Verification items for the finished model (mm, model axes). Round coordinates to 2 decimals unless told otherwise and drop trailing zeros. Loops run counter-clockwise (first coordinate to the right, second up) from the corner with the lowest first, then second, coordinate; pieces in that order, holes last. Notation, with made-up numbers: M -31,8.5 L 6,8.5 A20 cw 6,12.5 Z; hole C 22.5,36.25 d9. An arc over 180 degrees is marked long. One line per item, written item: value.
from build123d import *

# Parameters (mm, degrees)
F0_W     = 50
F0_H     = 20
F1_DEPTH = 114
F3_D     = 5
F3_DEPTH = 20.6
F3_TIP   = 1.5021515476
F5_D     = 10
F5_DEPTH = 42
F5_TIP   = 3.0043030951
F6_R     = 2


with BuildPart() as f1:
    # F0 (on Top) → F1 (new body)
    with BuildSketch(Plane.XY):
        Rectangle(F0_W, F0_H)
    extrude(amount=F1_DEPTH)

    # F3
    with Locations(Plane.XY.offset(114)):
        with Locations((-15, 0), (15, 0)):
            Hole(F3_D / 2, depth=F3_DEPTH)
            with Locations((0, 0, -(F3_DEPTH + F3_TIP / 2))):  # 118° drill point
                Cone(0, F3_D / 2, F3_TIP, mode=Mode.SUBTRACT)

    # F5
    with Locations(Plane(origin=(0, 0, 0), x_dir=(1, 0, 0), z_dir=(0, 0, -1))):
        with Locations((-15, 0), (15, 0)):
            Hole(F5_D / 2, depth=F5_DEPTH)
            with Locations((0, 0, -(F5_DEPTH + F5_TIP / 2))):  # 118° drill point
                Cone(0, F5_D / 2, F5_TIP, mode=Mode.SUBTRACT)

    # F6
    f6_edges = [f1.edges().sort_by_distance(p)[0] for p in [
        (25, -10, 57),
        (-25, -10, 57),
        (-25, 10, 57),
        (25, 10, 57),
    ]]
    fillet(f6_edges, radius=F6_R)


solid = f1.part
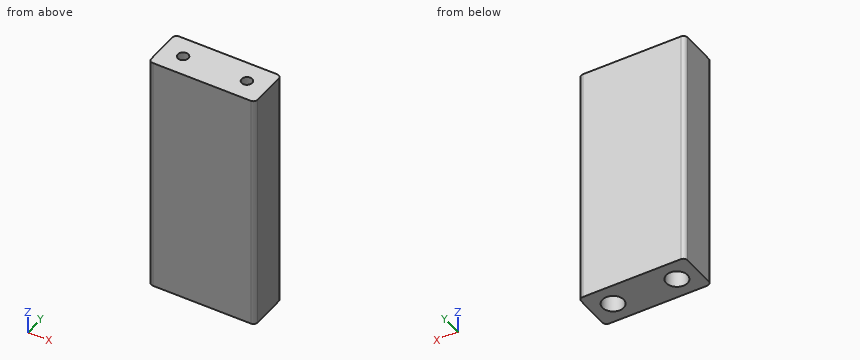
(1) Depth check by flat-ended pin: pin 1 Ø3 at (x, y) = (-15, 0) entering from +Z; pin 2 Ø4 at (x, y) = (15, 0) entering from -Z; pin 3 Ø6 at (x, y) = (-15, 0) entering from -Z. Enter the tip coordinate at first touch or a pass-through.
Completed:
pin 1: stops at z = 92.8
pin 2: stops at z = 43.8
pin 3: stops at z = 43.2
(2) Sectioned sample at A-A on z = 100. Enter the section's corners in (x, y), and give its area (3 significant figures).
Completed:
outline: M -25,-8 A2 ccw -23,-10 L 23,-10 A2 ccw 25,-8 L 25,8 A2 ccw 23,10 L -23,10 A2 ccw -25,8 Z; hole C -15,0 d5; hole C 15,0 d5
area: 957 mm^2
(3) Thickness scan on L1, parallel to X at y = 0, z = 103.5; L2, parallel to X at y = 0.5, z = 38; L3, parallel to Y at x = 15, z = 102. Record the ranges inside material, lowest first. Write a range as from..to.
Completed:
L1: x = -25..-17.5, -12.5..12.5, 17.5..25
L2: x = -25..-19.97, -10.03..10.03, 19.97..25
L3: y = -10..-2.5, 2.5..10
